The model under review builds one solid part; all positions refer to its coordinate system, in mm. A direction names the side the tool comes from. Coordinates: 2 decimals unless noted, no trailing zeros. Loops run counter-clockwise (first coordinate to the right, second up) from the corner with the lowest first, then second, coordinate; pieces in that order, holes last. Notation, with made-up numbers: M 14.5,-35 L 62.5,-35 A21 cw 62.5,-16 Z; hole C 42.5,69 d8. An arc over 180 degrees is marked long. Use CSV: the item, a comma, the result in double quotes. Start each with the question number.
1. Tool access review of faces 1 (the cylindrical face through (116.3, 3.3, -0.1)), 2 (the flat face through (66, 73.46, -6)), 3 (the flat face through (83, -1, 19)): name each direction out of +Z, -Z, +X, -X, +Y, -Y from which nothing blocks a thin tool from reaching the whole face with its end or side.
2. Add section A-A, the plane z = 16.5. Write out the cut boundary in (x, y).
3. Add section D-D, the plane x = 118. Write out the cut boundary in (y, z), then the cut area to 3 significant figures.
4. Draft analysis for pull direction Y (two halves, no side actions). For faces 4 (the flat face through (66, 90, 7)), 5 (the cylindrical face through (-4.609, -4.297, 5.689)), 6 (the flat face through (-5.75, 46, 6)), state which applies: +Y half, -Y half, draft (parallel to the pull), parting line (faces both ways), or undercut.
5. Add section C-C, the plane y = 24. Write out the cut boundary in (x, z), then the cut area to 3 significant figures.
6. Add section B-B, the plane x = 60.5. Write out the cut boundary in (y, z).
7. Clearance check with flat-ended pins moving along their axes: P1, Ø6.5, axis at x = 113.5, y = 85.5, coming from the +Z side; P2, Ø11, axis at x = 0.5, y = 22.5, coming from the +Z side; P3, Ø1, axis at y = 66, z = 4, coming from the -X side. State where each tip first meets the part, or that it passes through.
8. For L1, parallel to Y at x = 51, z = 2; L2, parallel to X at y = 58, z = 15.75; L3, parallel to X at y = 4.5, z = -4.5, list the stretches that pass through material, from the lowest coordinate up.
from build123d import *

# Parameters (mm, degrees)
BOSS_EXTRU_1_DEPTH                             = 19
BOSS_EXTRU_1_DEPTH_BACK                        = 8
ESQUISSE1_W                                    = 133.5
ESQUISSE1_H                                    = 90
ENL_V_MAT_EXTRU_1_DEPTH                        = 47
ENL_V_MAT_EXTRU_1_DEPTH_BACK                   = 5
FRAISAGE_POUR_VIS_T_TE_FRAIS_E_M32_D           = 3.4
FRAISAGE_POUR_VIS_T_TE_FRAIS_E_M32_DEPTH       = 5
FRAISAGE_POUR_VIS_T_TE_FRAIS_E_M32_CSINK_D     = 6.3
FRAISAGE_POUR_VIS_T_TE_FRAIS_E_M32_CSINK_ANGLE = 90
FRAISAGE_POUR_VIS_T_TE_FRAIS_E_M32_TIP         = 1.021463052
ESQUISSE7_W                                    = 24.511286956
ESQUISSE7_H                                    = 10.008551301
ENL_V_MAT_EXTRU_2_DEPTH                        = 10
ESQUISSE8_W                                    = 24.723742657
ESQUISSE8_H                                    = 11.436875975
ENL_V_MAT_EXTRU_3_DEPTH                        = 10
ESQUISSE9_W                                    = 24.478686325
ESQUISSE9_H                                    = 9.877285249
ENL_V_MAT_EXTRU_4_DEPTH                        = 10
CONG_1_R                                       = 0.5
ESQUISSE10_R                                   = 3
BOSS_EXTRU_2_DEPTH                             = 10
ESQUISSE12_W                                   = 98.408714422
ESQUISSE12_H                                   = 55.172933086
ENL_V_MAT_EXTRU_5_DEPTH                        = 10


with BuildPart() as part:
    # EsquisseExterieur → Boss.-Extru.1 (new body, two sides)
    with BuildSketch(Plane.XY) as boss_extru_1_sk:
        with BuildLine():
            Line((-1.75, -5.5), (135.25, -5.5))
            ThreePointArc((135.25, -5.5), (138.078427125, -4.328427125), (139.25, -1.5))
            Line((139.25, -1.5), (139.25, 91.5))
            ThreePointArc((139.25, 91.5), (138.078427125, 94.328427125), (135.25, 95.5))
            Line((135.25, 95.5), (-1.75, 95.5))
            ThreePointArc((-1.75, 95.5), (-4.578427125, 94.328427125), (-5.75, 91.5))
            Line((-5.75, 91.5), (-5.75, -1.5))
            ThreePointArc((-5.75, -1.5), (-4.578427125, -4.328427125), (-1.75, -5.5))
        make_face()
    extrude(amount=BOSS_EXTRU_1_DEPTH)
    extrude(boss_extru_1_sk.sketch, amount=-BOSS_EXTRU_1_DEPTH_BACK)

    # Esquisse1 → Enlèv. mat.-Extru.1 (cut, two sides)
    with BuildSketch(Plane.XY) as enl_v_mat_extru_1_sk:
        with Locations((66.75, 45)):
            Rectangle(ESQUISSE1_W, ESQUISSE1_H)
    extrude(amount=ENL_V_MAT_EXTRU_1_DEPTH, mode=Mode.SUBTRACT)
    extrude(enl_v_mat_extru_1_sk.sketch, amount=-ENL_V_MAT_EXTRU_1_DEPTH_BACK, mode=Mode.SUBTRACT)

    # Fraisage pour vis à tête fraisée M32
    with Locations(Plane.XY.offset(-5)):
        with Locations((4.145138972, 84.443401206), (127.127377422, 84.443401206), (127.127377422, 4.415852319), (4.240996888, 4.415852319)):
            CounterSinkHole(FRAISAGE_POUR_VIS_T_TE_FRAIS_E_M32_D / 2, FRAISAGE_POUR_VIS_T_TE_FRAIS_E_M32_CSINK_D / 2, depth=FRAISAGE_POUR_VIS_T_TE_FRAIS_E_M32_DEPTH, counter_sink_angle=FRAISAGE_POUR_VIS_T_TE_FRAIS_E_M32_CSINK_ANGLE)
            with Locations((0, 0, -(FRAISAGE_POUR_VIS_T_TE_FRAIS_E_M32_DEPTH + FRAISAGE_POUR_VIS_T_TE_FRAIS_E_M32_TIP / 2))):  # 118° drill point
                Cone(0, FRAISAGE_POUR_VIS_T_TE_FRAIS_E_M32_D / 2, FRAISAGE_POUR_VIS_T_TE_FRAIS_E_M32_TIP, mode=Mode.SUBTRACT)

    # Esquisse7 → Enlèv. mat.-Extru.2 (cut)
    with BuildSketch(Plane.ZY.offset(5.75)):
        with Locations((6.744356522, 65.353288209)):
            Rectangle(ESQUISSE7_W, ESQUISSE7_H)
    extrude(amount=-ENL_V_MAT_EXTRU_2_DEPTH, mode=Mode.SUBTRACT)

    # Esquisse8 → Enlèv. mat.-Extru.3 (cut)
    with BuildSketch(Plane.ZY.offset(5.75)):
        with Locations((6.638128671, 20.678831333)):
            Rectangle(ESQUISSE8_W, ESQUISSE8_H)
    extrude(amount=-ENL_V_MAT_EXTRU_3_DEPTH, mode=Mode.SUBTRACT)

    # Esquisse9 → Enlèv. mat.-Extru.4 (cut)
    with BuildSketch(Plane(origin=(139.25, 0, 0), x_dir=(0, 0, -1), z_dir=(1, 0, 0))):
        with Locations((-6.760656838, 73.668720261)):
            Rectangle(ESQUISSE9_W, ESQUISSE9_H)
    extrude(amount=-ENL_V_MAT_EXTRU_4_DEPTH, mode=Mode.SUBTRACT)

    # Congé1
    cong_1_edges = [part.edges().sort_by_distance(p)[0] for p in [
        (0, 7.480196672, 19),
        (133.5, 84.303681443, 19),
        (66.75, 90, 19),
        (133.5, 34.365038818, 19),
        (66.75, 0, 19),
        (0, 80.17878193, 19),
        (0, 43.373140939, 19),
    ]]
    fillet(cong_1_edges, radius=CONG_1_R)

    # Esquisse10 → Boss.-Extru.2 (add)
    with BuildSketch(Plane.XY.offset(-5)):
        with Locations((17.770805857, 84.443401206)):
            Circle(ESQUISSE10_R)
        with Locations((113.513450355, 84.443401206)):
            Circle(ESQUISSE10_R)
        with Locations((17.770805857, 4.415852319)):
            Circle(ESQUISSE10_R)
        with Locations((113.513450355, 4.415852319)):
            Circle(ESQUISSE10_R)
    extrude(amount=BOSS_EXTRU_2_DEPTH)

    # Esquisse12 → Enlèv. mat.-Extru.5 (cut)
    with BuildSketch(Plane.XY.offset(-5)):
        with Locations((66.458849957, 45.873450128)):
            Rectangle(ESQUISSE12_W, ESQUISSE12_H)
    extrude(amount=-ENL_V_MAT_EXTRU_5_DEPTH, mode=Mode.SUBTRACT)


solid = part.part
Computed:
1,face 1,"+Z"
1,face 2,"+Z, -Z"
1,face 3,"+Z, +X, -X, +Y, -Y"
2,outline,"M -5.75,-1.5 A4 ccw -1.75,-5.5 L 135.25,-5.5 A4 ccw 139.25,-1.5 L 139.25,68.73 L 133.5,68.73 L 133.5,0 L 0,0 L 0,14.96 L -5.75,14.96 Z; M -5.75,26.4 L 0,26.4 L 0,60.35 L -5.75,60.35 Z; M -5.75,70.36 L 0,70.36 L 0,90 L 133.5,90 L 133.5,78.61 L 139.25,78.61 L 139.25,91.5 A4 ccw 135.25,95.5 L -1.75,95.5 A4 ccw -5.75,91.5 Z"
3,outline,"M -5.5,-8 L 95.5,-8 L 95.5,19 L 90.5,19 A0.5 ccw 90,18.5 L 90,-5 L 0,-5 L 0,18.5 A0.5 ccw -0.5,19 L -5.5,19 Z"
3,area,"567 mm^2"
4,face 4,"undercut"
4,face 5,"-Y half"
4,face 6,"draft"
5,outline,"M -5.75,-8 L 17.25,-8 L 17.25,-5 L 4.25,-5 L 4.25,-5.72 L -5.75,-5.72 Z; M 115.66,-8 L 139.25,-8 L 139.25,19 L 134,19 A0.5 ccw 133.5,18.5 L 133.5,-5 L 115.66,-5 Z"
5,area,"270 mm^2"
6,outline,"M -5.5,-8 L 18.29,-8 L 18.29,-5 L 0,-5 L 0,18.5 A0.5 ccw -0.5,19 L -5.5,19 Z; M 73.46,-8 L 95.5,-8 L 95.5,19 L 90.5,19 A0.5 ccw 90,18.5 L 90,-5 L 73.46,-5 Z"
7,P1,"stops at z = 5"
7,P2,"stops at z = 19"
7,P3,"stops at x = 133.5"
8,L1,"y = -5.5 to 0, 90 to 95.5"
8,L2,"x = -5.75 to 0, 133.5 to 139.25"
8,L3,"x = -5.75 to 0, 14.77 to 20.77, 110.51 to 116.51, 133.5 to 139.25"
